The listing builds one solid part. Answer for the finished solid, in the listing's coordinates (mm). A direction names the side the tool comes from. Coordinates: 2 decimals unless noted, no trailing zeros.
```python
from build123d import *

# Parameters (mm, degrees)
SKETCH1_W                 = 67.2338
SKETCH1_H                 = 48.641
BOSS_EXTRUDE1_DEPTH       = 1.1303
F_3_0MM_DOWEL_HOLE1_D     = 3
SKETCH5_R                 = 5
BOSS_EXTRUDE2_DEPTH       = 17
FILLET1_R                 = 0.5
SKETCH6_W                 = 43
SKETCH6_H                 = 10
BOSS_EXTRUDE3_DEPTH       = 25
SKETCH7_W                 = 2.2
SKETCH7_H                 = 8.35
SKETCH7_W_2               = 2.85
CUT_EXTRUDE1_DEPTH        = 25
SKETCH8_W                 = 7.75
SKETCH8_H                 = 9.9
BOSS_EXTRUDE4_DEPTH       = 10
CHAMFER1_SIZE             = 1
CHAMFER1_SIZE2            = 3.732050808
CHAMFER1_OF_MIRROR2_SIZE2 = 1
CHAMFER1_OF_MIRROR2_SIZE  = 3.732050808


with BuildPart() as part:
    # Sketch1 → Boss-Extrude1 (new body)
    with BuildSketch(Plane(origin=(0, 0, 0), x_dir=(1, 0, 0), z_dir=(0, 1, 0))):
        Rectangle(SKETCH1_W, SKETCH1_H)
    extrude(amount=BOSS_EXTRUDE1_DEPTH)

    # Ø3.0mm Dowel Hole1 (through all)
    with Locations(Plane(origin=(0, 1.1303, 0), x_dir=(1, 0, 0), z_dir=(0, 1, 0))):
        with Locations((-27.94, -19.05), (-27.94, 19.05), (27.94, 19.05), (27.94, -19.05)):
            Hole(F_3_0MM_DOWEL_HOLE1_D / 2)

    # Sketch5 → Boss-Extrude2 (add)
    with BuildSketch(Plane(origin=(0, 1.1303, 0), x_dir=(1, 0, 0), z_dir=(0, 1, 0))):
        with Locations((-26.9875, 10.668)):
            Circle(SKETCH5_R)
        with Locations((-26.9875, -10.668)):
            Circle(SKETCH5_R)
        with Locations((26.9875, 10.668)):
            Circle(SKETCH5_R)
        with Locations((26.9875, -10.668)):
            Circle(SKETCH5_R)
    extrude(amount=BOSS_EXTRUDE2_DEPTH)

    # Fillet1
    fillet1_edges = [part.edges().sort_by_distance(p)[0] for p in [
        (-31.9875, 18.1303, -10.668),
        (-31.9875, 18.1303, 10.668),
        (21.9875, 18.1303, -10.668),
        (21.9875, 18.1303, 10.668),
    ]]
    fillet(fillet1_edges, radius=FILLET1_R)

    # Sketch6 → Boss-Extrude3 (add)
    with BuildSketch(Plane(origin=(0, 1.1303, 0), x_dir=(1, 0, 0), z_dir=(0, 1, 0))):
        with Locations((0, 18.25)):
            Rectangle(SKETCH6_W, SKETCH6_H)
    boss_extrude3 = extrude(amount=BOSS_EXTRUDE3_DEPTH)

    # Sketch7 → Cut-Extrude1 (cut)
    with BuildSketch(Plane(origin=(0, 26.1303, 0), x_dir=(1, 0, 0), z_dir=(0, 1, 0))):
        with Locations((-19.1, 19.075)):
            Rectangle(SKETCH7_W, SKETCH7_H)
        with Locations((-15.575, 19.075)):
            Rectangle(SKETCH7_W_2, SKETCH7_H)
        with Locations((19.1, 19.075)):
            Rectangle(SKETCH7_W, SKETCH7_H)
        with Locations((-11.675, 19.075)):
            Rectangle(SKETCH7_W_2, SKETCH7_H)
        with Locations((-7.775, 19.075)):
            Rectangle(SKETCH7_W_2, SKETCH7_H)
        with Locations((-3.875, 19.075)):
            Rectangle(SKETCH7_W_2, SKETCH7_H)
        with Locations((0.025, 19.075)):
            Rectangle(SKETCH7_W_2, SKETCH7_H)
        with Locations((3.925, 19.075)):
            Rectangle(SKETCH7_W_2, SKETCH7_H)
        with Locations((7.825, 19.075)):
            Rectangle(SKETCH7_W_2, SKETCH7_H)
        with Locations((11.725, 19.075)):
            Rectangle(SKETCH7_W_2, SKETCH7_H)
        with Locations((15.625, 19.075)):
            Rectangle(SKETCH7_W_2, SKETCH7_H)
    cut_extrude1 = extrude(amount=-CUT_EXTRUDE1_DEPTH, mode=Mode.SUBTRACT)

    # Mirror1: Boss-Extrude3, Cut-Extrude1 across plane
    add(boss_extrude3.mirror(Plane.XY))
    add(cut_extrude1.mirror(Plane.XY), mode=Mode.SUBTRACT)

    # Sketch8 → Boss-Extrude4 (add)
    with BuildSketch(Plane(origin=(0, 1.1303, 0), x_dir=(1, 0, 0), z_dir=(0, 1, 0))):
        with Locations((28.275, 0)):
            Rectangle(SKETCH8_W, SKETCH8_H)
    boss_extrude4 = extrude(amount=BOSS_EXTRUDE4_DEPTH)

    # Chamfer1
    chamfer1_edges = [part.edges().sort_by_distance(p)[0] for p in [
        (24.4, 11.1303, 0),
        (32.15, 11.1303, 0),
    ]]
    chamfer1_side = [part.faces().sort_by_distance(p)[0] for p in [
        (28.275, 11.1303, 0),
    ]]
    chamfer(chamfer1_edges, length=CHAMFER1_SIZE, length2=CHAMFER1_SIZE2, reference=chamfer1_side[0])

    # Mirror2: Boss-Extrude4 across plane
    add(boss_extrude4.mirror(Plane(origin=(0, 0, 0), x_dir=(0, 0, 1), z_dir=(1, 0, 0))))

    # Chamfer1 of Mirror2
    chamfer1_of_mirror2_edges = [part.edges().sort_by_distance(p)[0] for p in [
        (-24.4, 11.1303, 0),
        (-32.15, 11.1303, 0),
    ]]
    chamfer(chamfer1_of_mirror2_edges, length=CHAMFER1_OF_MIRROR2_SIZE, length2=CHAMFER1_OF_MIRROR2_SIZE2)


solid = part.part
```
(1) Each of these flat-tipped pins is pushed along its axis until it touches: pin 1 Ø6.5 at (y, z) = (13, 17.5) entering from -X; pin 2 Ø2.5 at (x, y) = (-8, 15.5) entering from -Z; pin 3 Ø0.9 at (x, y) = (-11.5, 19.5) entering from -Z; pin 4 Ø4 at (x, y) = (-24.5, 23.5) entering from +Z. Where does it stop, or does it pass through?
(2) The mould has two halves that part along Z. Classify faces 1 (the face through (29.44, 0.56, 18.98)), 2 (the face through (4, 26.13, -14)), 3 (the face through (-19, 14, 14.9)), 4 (the face through (-16, 14, -14.9)): released by +Z, released by -Z, zero draft, split by the parting line, or undercut.
(3) Find section A-A (z = 19.05). Give the number of separate pieces and of enclosed holes in the cut face, and give its area (3 significant figures).
(4) For faces 5 (the face through (-9.2, 14, -19)), 6 (the face through (-16, 14, 14.9)), determine the directions among +Z, -Z, +X, -X, +Y, -Y from which every point of the face is accessible in a straight line to the end or side of a thin tool.
(5) Consider line 1 (Z direction, x = 27.94, y = 0.35); line 2 (X direction, y = 0.8, z = 19.05); line 3 (X direction, y = 7.25, z = -1). Determine where each line is inside the solid, lowest interval first.
Findings below:
1. pin 1: stops at x = -30.48
1. pin 2: stops at z = -23.25
1. pin 3: stops at z = -14.9
1. pin 4: passes through
2. face 1: undercut
2. face 2: zero draft
2. face 3: released by +Z
2. face 4: released by -Z
3. separate pieces: 3
3. enclosed holes: 0
3. area: 393 mm2
4. face 5: -Z, +Y
4. face 6: +Z, +Y
5. line 1: z = -24.32 to -20.55, -17.55 to 17.55, 20.55 to 24.32
5. line 2: x = -33.62 to -29.44, -26.44 to 26.44, 29.44 to 33.62
5. line 3: x = -32.15 to -24.4, 24.4 to 32.15
